```python
from build123d import *

# Parameters (mm, degrees)
BOSS_EXTRUDE1_DEPTH = 2
SKETCH2_R           = 7.5
BOSS_EXTRUDE2_DEPTH = 2
SKETCH3_R           = 2.5
BOSS_EXTRUDE3_DEPTH = 10
SKETCH4_R           = 1
BOSS_EXTRUDE4_DEPTH = 20
SKETCH5_R           = 1.5
BOSS_EXTRUDE5_DEPTH = 5
BOSS_EXTRUDE6_DEPTH = 11
SKETCH7_R           = 1
BOSS_EXTRUDE7_DEPTH = 10
CHAMFER1_SIZE       = 1


with BuildPart() as part:
    # Sketch1 → Boss-Extrude1 (new body)
    with BuildSketch(Plane.XY):
        Polygon((7.397125851, -4.5036129), (7.598806105, 4.154292452), (0.201680255, 8.657905351), (-7.397125851, 4.5036129), (-7.598806105, -4.154292452), (-0.201680255, -8.657905351), align=None)
    extrude(amount=-BOSS_EXTRUDE1_DEPTH)

    # Sketch2 → Boss-Extrude2 (add)
    with BuildSketch(Plane.XY):
        with Locations(Location((0, 0, 0), (0, 0, 178.665573541))):
            Circle(SKETCH2_R)
    extrude(amount=BOSS_EXTRUDE2_DEPTH)

    # Sketch3 → Boss-Extrude3 (add)
    with BuildSketch(Plane.XY.offset(2)):
        Circle(SKETCH3_R)
    extrude(amount=BOSS_EXTRUDE3_DEPTH)

    # Sketch4 → Boss-Extrude4 (add)
    with BuildSketch(Plane.XY.offset(12)):
        Circle(SKETCH4_R)
    extrude(amount=BOSS_EXTRUDE4_DEPTH)

    # Sketch5 → Boss-Extrude5 (add)
    with BuildSketch(Plane.XY.offset(32)):
        Circle(SKETCH5_R)
    extrude(amount=BOSS_EXTRUDE5_DEPTH)

    # Sketch6 → Boss-Extrude6 (add)
    with BuildSketch(Plane(origin=(0, 0, -2), x_dir=(-1, 0, 0), z_dir=(0, 0, -1))):
        Polygon((-7.598806105, 4.154292452), (-0.201680255, 8.657905351), (7.397125851, 4.5036129), (7.598806105, -4.154292452), (0.201680255, -8.657905351), (-7.397125851, -4.5036129), align=None)
    extrude(amount=BOSS_EXTRUDE6_DEPTH)

    # Sketch7 → Boss-Extrude7 (add)
    with BuildSketch(Plane(origin=(0, 0, -13), x_dir=(-1, 0, 0), z_dir=(0, 0, -1))):
        with BuildLine():
            Line((-13.7, 16), (13.7, 16))
            ThreePointArc((13.7, 16), (15.326345597, 15.326345597), (16, 13.7))
            Line((16, 13.7), (16, -13.7))
            ThreePointArc((16, -13.7), (15.326345597, -15.326345597), (13.7, -16))
            Line((13.7, -16), (-13.7, -16))
            ThreePointArc((-13.7, -16), (-15.326345597, -15.326345597), (-16, -13.7))
            Line((-16, -13.7), (-16, 13.7))
            ThreePointArc((-16, 13.7), (-15.326345597, 15.326345597), (-13.7, 16))
        make_face()
        with Locations((-13.5, 13.5)):
            Circle(SKETCH7_R, mode=Mode.SUBTRACT)
        with Locations((13.5, 13.5)):
            Circle(SKETCH7_R, mode=Mode.SUBTRACT)
        with Locations((13.5, -13.5)):
            Circle(SKETCH7_R, mode=Mode.SUBTRACT)
        with Locations((-13.5, -13.5)):
            Circle(SKETCH7_R, mode=Mode.SUBTRACT)
    extrude(amount=BOSS_EXTRUDE7_DEPTH)

    # Chamfer1
    chamfer1_edges = [part.edges().sort_by_distance(p)[0] for p in [
        (-12.5, -13.5, -13),
        (14.5, 13.5, -13),
        (-12.5, 13.5, -13),
        (14.5, -13.5, -13),
    ]]
    chamfer(chamfer1_edges, length=CHAMFER1_SIZE)


solid = part.part
```
CAD build for the part. Positions are in the model's coordinates, mm. A direction names the side the tool comes from. Round coordinates to 2 decimals unless told otherwise and drop trailing zeros. Order: outer loops, then holes, each group sorted by start corner. A loop starts at its lowest first (then second) coordinate and runs counter-clockwise, first axis right, second up. Notation, with made-up numbers: (67.25, 2) -> (124.25, 2) arc R33 cw to (124.25, 31) -> close; hole circle Ø4 at (67.25, -26.75). An arc over 180 degrees is marked (long way). One line per question, with ' | ' between items.
Q1. Which spindle directions (+Z, -Z, +X, -X, +Y, -Y) get a long thin tool onto all of the face, cutting with end or side? Do faces 1 (the flat face through (-7, -4, 0)), 2 (the flat face through (3.545, -6.61, -6.409)), 3 (the cylindrical face through (-0.54, -2.44, 6.93)), 4 (the flat face through (7, 4, 0)). Say none if no direction does.
Completed:
face 1: +Z, -X, -Y | face 2: +Z, +X, -Y | face 3: +Z | face 4: +Z, +X, +Y
Q2. Slice it at A-A (z = -16.5). Write the cut outline in (x, y), then the cut area to 3 significant figures.
Completed:
outline: (-16, -13.7) arc R2.3 ccw to (-13.7, -16) -> (13.7, -16) arc R2.3 ccw to (16, -13.7) -> (16, 13.7) arc R2.3 ccw to (13.7, 16) -> (-13.7, 16) arc R2.3 ccw to (-16, 13.7) -> close; hole circle Ø2 at (-13.5, -13.5); hole circle Ø2 at (-13.5, 13.5); hole circle Ø2 at (13.5, -13.5); hole circle Ø2 at (13.5, 13.5) | area: 1,010 mm^2
Q3. Slice it at C-C (x = -10). Write the cut outline in (y, z), then the cut area to 3 significant figures.
Completed:
outline: (-16, -23) -> (16, -23) -> (16, -13) -> (-16, -13) -> close | area: 320 mm^2
Q4. Two-plate mould, pull along X, no slides. Class faces 5 (the flat face through (0, -16, -18)), 6 (the cylindrical face through (-13.96, 12.61, -18.44)), 7 (the flat face through (-3.952, -6.375, -6.409)): released by +X, released by -X, zero draft, split by the parting line, or undercut.
Completed:
face 5: zero draft | face 6: undercut | face 7: released by -X
Q5. Drop flat-ended pins along their axis: pin 1 (4 mm diameter, centred on x = -4.5, z = 16.5, fed in from +Y); pin 2 (4 mm diameter, centred on x = -6, y = -3.5, fed in from +Z). Give the stop position or say it passes through.
Completed:
pin 1: passes through | pin 2: stops at z = 2
Q6. Probe probe 1 along Y at (x, z) = (13.5, -16); probe 2 along X at (y, z) = (-13, -19); probe 3 along Z at (x, y) = (11.5, -5.5). List the from-to ranges inside material, lowest first.
Completed:
probe 1: y = -16 to -14.5, -12.5 to 12.5, 14.5 to 16 | probe 2: x = -16 to -14.37, -12.63 to 12.63, 14.37 to 16 | probe 3: z = -23 to -13
Q7. Slice it at B-B (z = -2.5). Write the cut outline in (x, y).
Completed:
outline: (-7.6, -4.15) -> (-0.2, -8.66) -> (7.4, -4.5) -> (7.6, 4.15) -> (0.2, 8.66) -> (-7.4, 4.5) -> close
